Here's how the part is built. I have some questions about the finished solid (model axes, mm). A direction names the side the tool comes from. Coordinates: 2 decimals unless noted, no trailing zeros. Write each loop counter-clockwise with the first axis right and the second up, starting at its lowest first coordinate (ties: lowest second). Pieces come first, ordered by that corner, then holes.
Item 1: For faces 1 (the face through (10.3, 23.93, 15.7)), 2 (the face through (11.786, 22.098, 14.087)), which set-ups out of +Z, -Z, +X, -X, +Y, -Y let a thin tool reach every point of the face, with its end or its side?
Item 2: If we mould it in two halves opening along Y, with no side actions, what happens to faces 3 (the face through (0, 40, 3.175)), 4 (the face through (0, 39, 0)), 5 (the face through (-12.12, 22.726, 14.087))? For each: pulls with the +Y half, pulls with the -Y half, needs draft (parallel to the pull), parting line crosses it, or undercut.
Item 3: Please list where these lines run through material, in increasing order: line 1 (X direction, y = 50.8, z = 15); line 2 (X direction, y = 56, z = 5.5); line 3 (Z direction, x = -1, y = 25.5) (3 decimals).
Item 4: I'm going to push flat-ended pins straight in: P1, Ø1, axis at x = 17.5, y = 48.5, coming from the +Z side (3 decimals); P2, Ø5, axis at x = 3.5, z = 12.5, coming from the -Y side (3 decimals); P3, Ø3, axis at x = -6, z = 6, coming from the -Y side. Where does each tip first touch, or does it pass through?
Item 5: I want a section at A-A (z = 19.5). Please give me the cut outline in (x, y) (1 decimal), and give its area (3 significant figures).
Item 6: I want a section at B-B (x = -8). Please give me the cut outline in (y, z) (3 decimals).
Item 7: I want a section at C-C (y = 33). Please give me the cut outline in (x, z) (3 decimals), and give its area (3 significant figures).
from build123d import *

# Parameters (mm, degrees)
F1_DEPTH = 3.175
F3_DEPTH = 25.4


with BuildPart() as f1:
    # F0 (on Top) → F1 (new body)
    with BuildSketch(Plane.XY):
        with BuildLine():
            Line((0.205414, 53.074933), (-0.205414, 53.074933))
            ThreePointArc((-0.205414, 53.074933), (-16.875716, 62.79389), (-23.905882, 44.823529))
            Line((-23.905882, 44.823529), (0, 0))
            Line((0, 0), (23.905882, 44.823529))
            ThreePointArc((23.905882, 44.823529), (16.875716, 62.79389), (0.205414, 53.074933))
        make_face()
    extrude(amount=F1_DEPTH)

    # F2 (on face) → F3 (join)
    with BuildSketch(Plane.XY.offset(3.175)):
        with BuildLine():
            ThreePointArc((23.905882, 44.823529), (16.875716, 62.79389), (0.205414, 53.074933))
            Line((0.205414, 53.074933), (-0.205414, 53.074933))
            ThreePointArc((-0.205414, 53.074933), (-16.875716, 62.79389), (-23.905882, 44.823529))
            Line((-23.905882, 44.823529), (0, 0))
            Line((0, 0), (23.905882, 44.823529))
        make_face()
        with BuildLine():
            ThreePointArc((-20.315473, 42.707274), (-17.421546, 60.859556), (-1.608783, 51.487433))
            Line((-1.608783, 51.487433), (1.608783, 51.487433))
            ThreePointArc((1.608783, 51.487433), (17.421546, 60.859556), (20.315473, 42.707274))
            Line((20.315473, 42.707274), (0, 4.615761))
            Line((0, 4.615761), (-20.315473, 42.707274))
        make_face(mode=Mode.SUBTRACT)
    extrude(amount=F3_DEPTH)


solid = f1.part
Answer:
1. face 1: +Z
1. face 2: +Z, -Z, +X, -Y
2. face 3: undercut
2. face 4: needs draft
2. face 5: pulls with the -Y half
3. line 1: x = -25.4 to -23.81, 23.81 to 25.4
3. line 2: x = -24.29 to -22.52, -2.88 to -1.11, 1.11 to 2.88, 22.52 to 24.29
3. line 3: z = 0 to 3.175
4. P1: stops at z = 3.175
4. P2: stops at y = 1.875
4. P3: stops at y = 8.44
5. outline: (-23.9, 44.8) - (0, 0) - (23.9, 44.8) arc R12.7 ccw (long way) to (0.2, 53.1) - (-0.2, 53.1) arc R12.7 ccw (long way) to start; hole (-20.3, 42.7) - (0, 4.6) - (20.3, 42.7) arc R11.1 ccw (long way) to (1.6, 51.5) - (-1.6, 51.5) arc R11.1 ccw (long way) to start
5. area: 344 mm2
6. outline: (15, 0) - (62.598, 0) - (62.598, 28.575) - (60.87, 28.575) - (60.87, 3.175) - (19.616, 3.175) - (19.616, 28.575) - (15, 28.575) - close
7. outline: (-17.6, 0) - (17.6, 0) - (17.6, 28.575) - (15.138, 28.575) - (15.138, 3.175) - (-15.138, 3.175) - (-15.138, 28.575) - (-17.6, 28.575) - close
7. area: 237 mm2
